```python
from build123d import *

# Parameters (mm, degrees)
BOSS_EXTRUDE1_DEPTH = 3.4036


with BuildPart() as part:
    # Sketch1 → Boss-Extrude1 (new body)
    with BuildSketch(Plane.XY):
        Polygon((8548.865297466, 2983.807539807), (8548.865297466, 2943.218339807), (8542.515297466, 2943.218339807), (8542.515297466, 2930.518339807), (8694.915297466, 2930.518339807), (8694.915297466, 2943.218339807), (8688.565297466, 2943.218339807), (8688.565297466, 2983.807539807), (8694.915297466, 2983.807539807), (8694.915297466, 2996.507539807), (8542.515297466, 2996.507539807), (8542.515297466, 2983.807539807), align=None)
        with BuildLine():
            ThreePointArc((8571.090297466, 2946.393339807), (8566.600169406, 2948.253211746), (8564.740297466, 2952.743339807))
            Line((8564.740297466, 2952.743339807), (8564.740297466, 2974.282539807))
            ThreePointArc((8564.740297466, 2974.282539807), (8566.600169406, 2978.772667867), (8571.090297466, 2980.632539807))
            Line((8571.090297466, 2980.632539807), (8666.340297466, 2980.632539807))
            ThreePointArc((8666.340297466, 2980.632539807), (8670.830425527, 2978.772667867), (8672.690297466, 2974.282539807))
            Line((8672.690297466, 2974.282539807), (8672.690297466, 2952.743339807))
            ThreePointArc((8672.690297466, 2952.743339807), (8670.830425527, 2948.253211746), (8666.340297466, 2946.393339807))
            Line((8666.340297466, 2946.393339807), (8571.090297466, 2946.393339807))
        make_face(mode=Mode.SUBTRACT)
    extrude(amount=BOSS_EXTRUDE1_DEPTH)


solid = part.part
```
Check sheet for the modelled part. Datum: model origin and axes. Units: mm. A direction names the side the tool comes from. Round coordinates to 2 decimals unless told otherwise and drop trailing zeros. Order: outer loops, then holes, each group sorted by start corner. A loop starts at its lowest first (then second) coordinate and runs counter-clockwise, first axis right, second up. Notation, with made-up numbers: M 62,89 L 81,89 A9 cw 81,94 Z; hole C 88,27 d3. An arc over 180 degrees is marked long. Answer in a Markdown table with one row per item.
(1) Section check B-B on x = 8587.5. Record the boundary of the cut face in (y, z).
Findings:
| item | result |
|---|---|
| outline | M 2930.52,0 L 2946.39,0 L 2946.39,3.4 L 2930.52,3.4 Z; M 2980.63,0 L 2996.51,0 L 2996.51,3.4 L 2980.63,3.4 Z |
(2) Section check C-C on z = 1.45. Record the boundary of the cut face in (x, y), plus the area to 3 significant figures.
Findings:
| item | result |
|---|---|
| outline | M 8542.52,2930.52 L 8694.92,2930.52 L 8694.92,2943.22 L 8688.57,2943.22 L 8688.57,2983.81 L 8694.92,2983.81 L 8694.92,2996.51 L 8542.52,2996.51 L 8542.52,2983.81 L 8548.87,2983.81 L 8548.87,2943.22 L 8542.52,2943.22 Z; hole M 8564.74,2952.74 A6.35 ccw 8571.09,2946.39 L 8666.34,2946.39 A6.35 ccw 8672.69,2952.74 L 8672.69,2974.28 A6.35 ccw 8666.34,2980.63 L 8571.09,2980.63 A6.35 ccw 8564.74,2974.28 Z |
| area | 5,880 mm^2 |
(3) Material ranges on line 1 along Y through (x, z) = (8655, 3.1); line 2 along X through (y, z) = (2969.5, 2.3); line 3 along X through (y, z) = (2976, 2), recorded low to high. Write a range as from..to.
Findings:
| item | result |
|---|---|
| line 1 | y = 2930.52..2946.39, 2980.63..2996.51 |
| line 2 | x = 8548.87..8564.74, 8672.69..8688.57 |
| line 3 | x = 8548.87..8564.98, 8672.45..8688.57 |
(4) Draft check along X on faces 1 (the flat face through (8692, 2983.808, 2)), 2 (the flat face through (8548.865, 2964, 2)), 3 (the cylindrical face through (8670.88, 2948.303, 1.678)). Enter one of: +X half, -X half, draft (parallel to the pull), parting line (faces both ways), or undercut.
Findings:
| item | result |
|---|---|
| face 1 | draft |
| face 2 | -X half |
| face 3 | undercut |
(5) Gauge pin test, flat ends, axial feed: pin 1 (10 mm diameter, centred on x = 8627, y = 2955, fed in from -Z); pin 2 (1.7 mm diameter, centred on y = 2971.5, z = 2, fed in from +X); pin 3 (6 mm diameter, centred on x = 8651.5, y = 2947, fed in from +Z). Record the tip position at first contact, or that the pin passes through.
Findings:
| item | result |
|---|---|
| pin 1 | passes through |
| pin 2 | stops at x = 8688.57 |
| pin 3 | stops at z = 3.4 |
(6) Set-up check for faces 4 (the flat face through (8618, 2980.633, 2)), 5 (the flat face through (8546, 2983.808, 2)), 6 (the flat face through (8692, 2943.218, 2)): record each of +Z, -Z, +X, -X, +Y, -Y from which the full face is reachable in a straight line by a thin tool's end or side.
Findings:
| item | result |
|---|---|
| face 4 | +Z, -Z |
| face 5 | +Z, -Z, -X |
| face 6 | +Z, -Z, +X |
(7) Section check A-A on y = 2961. Record the boundary of the cut face in (x, z), plus the area to 3 significant figures.
Findings:
| item | result |
|---|---|
| outline | M 8548.87,0 L 8564.74,0 L 8564.74,3.4 L 8548.87,3.4 Z; M 8672.69,0 L 8688.57,0 L 8688.57,3.4 L 8672.69,3.4 Z |
| area | 108 mm^2 |
